Drawing for the job (mm, zero at the part's lowest x, y, z). Round coordinates to 2 decimals unless told otherwise and drop trailing zeros. Loops run counter-clockwise (first coordinate to the right, second up) from the corner with the lowest first, then second, coordinate; pieces in that order, holes last.
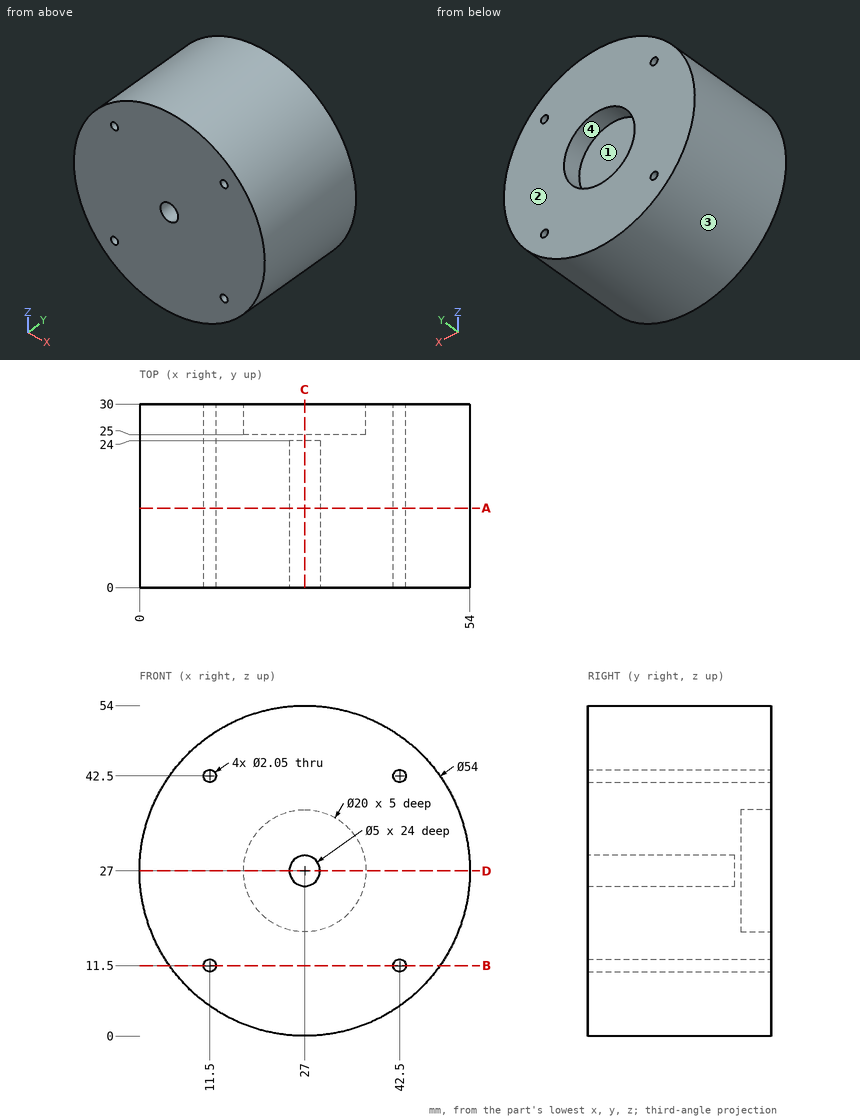
Q1. Probe line 1 (X direction, y = 18.25, z = 27); line 2 (Z direction, x = 12, y = 16); line 3 (X direction, y = 12.5, z = 42.5) (3 decimals). List the from-to ranges inside material, lowest first.
Q2. Slice it at B-B on z = 11.5. Give the cut face in (x, y) (3 decimals).
Q3. Slice it at A-A on y = 13. Give the cut face in (x, z) (3 decimals), plus the area to 3 significant figures.
Q4. Pull direction X, two halves, no side cores. Call the marked faces 1, 2, 3 and 4: pulls with the +X half, pulls with the -X half, needs draft (parallel to the pull), parting line crosses it, or undercut.
Q5. Flat gauge pins, fed straight in: P1, Ø5, axis at y = 19, z = 16.5, coming from the -X side; P2, Ø2, axis at y = 8, z = 44, coming from the +X side; P3, Ø2, axis at x = 22, y = 10.5, coming from the -Z side. Where does each tip first touch, or does it go through?
Q6. Slice it at C-C on x = 27. Give the cut face in (y, z), plus the area to 3 significant figures.
Q7. Slice it at D-D on z = 27. Give the cut face in (x, y).
Reply:
1. line 1: x = 0 to 24.5, 29.5 to 54
1. line 2: z = 4.55 to 10.61, 12.39 to 41.61, 43.39 to 49.45
1. line 3: x = 4.892 to 10.475, 12.525 to 41.475, 43.525 to 49.108
2. outline: (4.892, 0) - (10.475, 0) - (10.475, 30) - (4.892, 30) - close; (12.525, 0) - (41.475, 0) - (41.475, 30) - (12.525, 30) - close; (43.525, 0) - (49.108, 0) - (49.108, 30) - (43.525, 30) - close
3. outline: circle Ø54 at (27, 27); hole circle Ø2.05 at (11.5, 11.5); hole circle Ø2.05 at (11.5, 42.5); hole circle Ø5 at (27, 27); hole circle Ø2.05 at (42.5, 11.5); hole circle Ø2.05 at (42.5, 42.5)
3. area: 2,260 mm2
4. face 1: undercut
4. face 2: needs draft
4. face 3: parting line crosses it
4. face 4: undercut
5. P1: stops at x = 1.21
5. P2: stops at x = 48.75
5. P3: stops at z = 0.3
6. outline: (0, 0) - (30, 0) - (30, 17) - (25, 17) - (25, 37) - (30, 37) - (30, 54) - (0, 54) - (0, 29.5) - (24, 29.5) - (24, 24.5) - (0, 24.5) - close
6. area: 1,400 mm2
7. outline: (0, 0) - (24.5, 0) - (24.5, 24) - (29.5, 24) - (29.5, 0) - (54, 0) - (54, 30) - (37, 30) - (37, 25) - (17, 25) - (17, 30) - (0, 30) - close
